Input: dimensioned drawing with shaded views. Units: mm. Origin: part minimum x, y, z. A direction names the side the tool comes from. Give positions to 0.01 mm unless a question says otherwise; leave off trailing zeros. Loops run counter-clockwise (first coordinate to the right, second up) from the corner with the lowest first, then second, coordinate; pieces in that order, holes last. Notation, with made-up numbers: M -17,-23 L 19,-23 A19 ccw 19,-3 Z; hole C 64,33 d5. An arc over 180 degrees is marked long. Use CSV: the item, a comma, the result in double quotes. Start each with the question number.
Q1. Reachability of the marked faces 1 and 2 from +Z, -Z, +X, -X, +Y, -Y: full face, straight path, thin tool, end or side. Return the list, or none.
Q2. Section B-B, the plane x = 8.5. Output: boundary loops of the cut face in (y, z), plus the area to 3 significant figures.
Q3. Section C-C, the plane z = 23.5. Output: boundary loops of the cut face in (x, y).
Q4. Section A-A, the plane y = 6.35. Output: boundary loops of the cut face in (x, z), plus the area to 3 significant figures.
Q5. Material intervals for line 1 along Z through (x, y) = (1.5, 68.95); line 2 along Y through (x, z) = (1.05, 81.5); line 3 along Z through (x, y) = (8.75, 9.5), sorted ascending.
Q6. Section D-D, the plane y = 19.95. Output: boundary loops of the cut face in (x, z).
Q7. Pin query (flat end, axial travel): pin 1 (7 mm diameter, centred on x = 10.14, y = 6.35, fed in from +Z); pin 2 (4.5 mm diameter, centred on y = 68.95, z = 81.5, fed in from +X). Return the tip coordinate at first contact, or that it passes through.
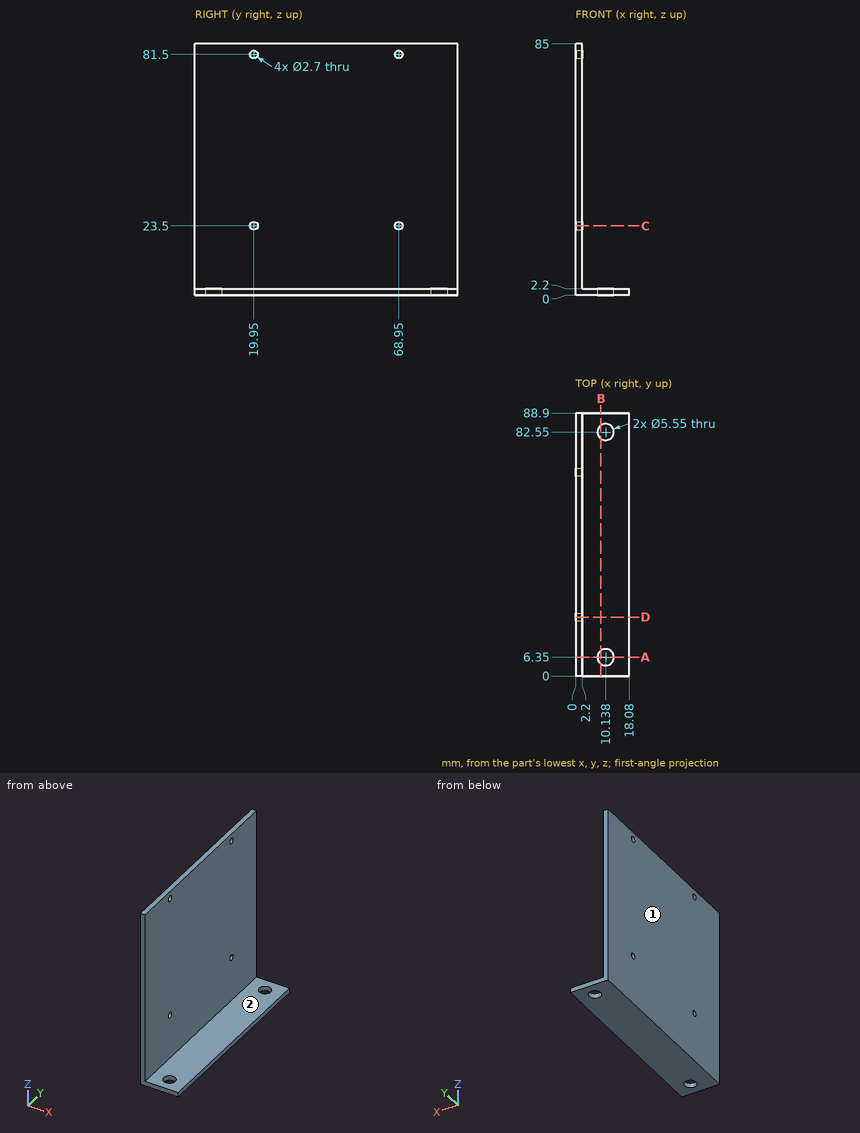
A:
1,face 1,"+Z, -Z, -X, +Y, -Y"
1,face 2,"+Z, +X, +Y, -Y"
2,outline,"M 0,0 L 4.11,0 L 4.11,2.2 L 0,2.2 Z; M 8.59,0 L 80.31,0 L 80.31,2.2 L 8.59,2.2 Z; M 84.79,0 L 88.9,0 L 88.9,2.2 L 84.79,2.2 Z"
2,area,"176 mm^2"
3,outline,"M 0,0 L 2.2,0 L 2.2,18.6 L 0,18.6 Z; M 0,21.3 L 2.2,21.3 L 2.2,67.6 L 0,67.6 Z; M 0,70.3 L 2.2,70.3 L 2.2,88.9 L 0,88.9 Z"
4,outline,"M 0,0 L 7.36,0 L 7.36,2.2 L 2.2,2.2 L 2.2,85 L 0,85 Z; M 12.91,0 L 18.08,0 L 18.08,2.2 L 12.91,2.2 Z"
4,area,"210 mm^2"
5,line 1,"0 to 22.15, 24.85 to 80.15, 82.85 to 85"
5,line 2,"0 to 18.6, 21.3 to 67.6, 70.3 to 88.9"
5,line 3,"0 to 2.2"
6,outline,"M 0,0 L 18.08,0 L 18.08,2.2 L 2.2,2.2 L 2.2,22.15 L 0,22.15 Z; M 0,24.85 L 2.2,24.85 L 2.2,80.15 L 0,80.15 Z; M 0,82.85 L 2.2,82.85 L 2.2,85 L 0,85 Z"
7,pin 1,"z = 2.2"
7,pin 2,"x = 2.2"
